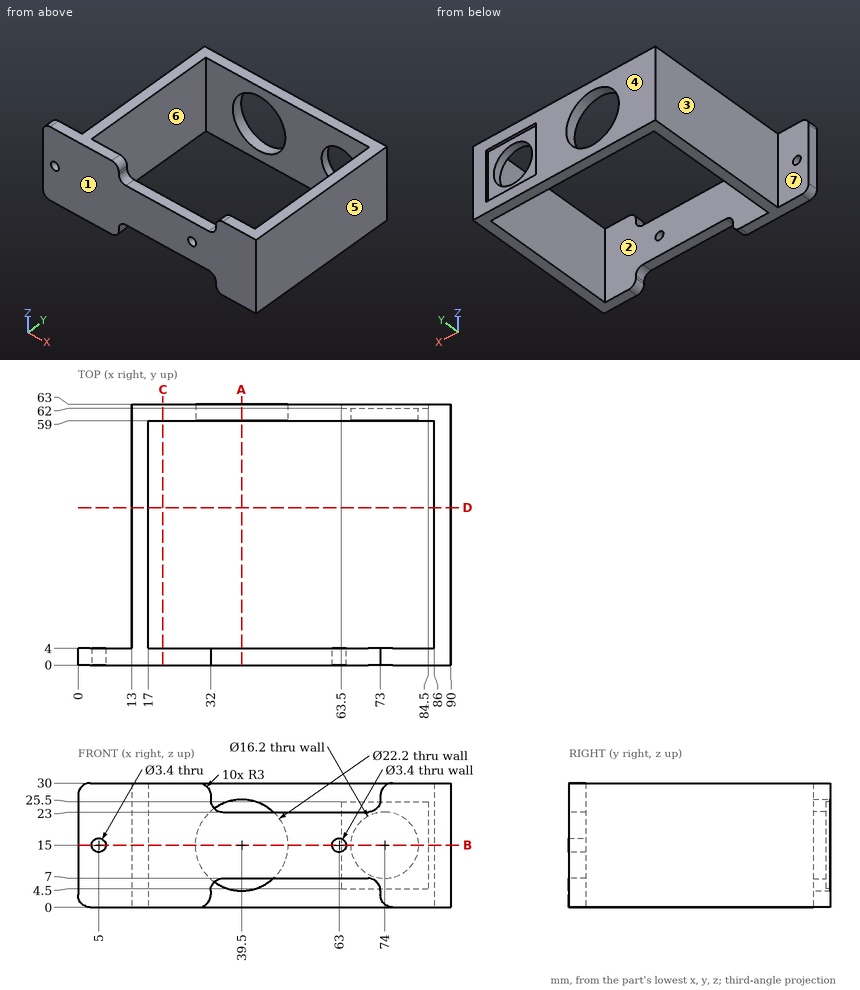
Here's the drawing with two shaded views (mm, measured from the low corner). I have some questions. A direction names the side the tool comes from. Coordinates: 2 decimals unless noted, no trailing zeros. Loops run counter-clockwise (first coordinate to the right, second up) from the corner with the lowest first, then second, coordinate; pieces in that order, holes last. Notation, with made-up numbers: (68, 70) -> (92, 70) arc R17 ccw to (92, 103) -> close; hole circle Ø3 at (65, 47.25). An arc over 180 degrees is marked (long way). Answer in a Markdown table with one row per item.
(1) Imagine slicing it at D-D (y = 38). List the corners of the cut face in (x, z) for me.
Results found:
| item | result |
|---|---|
| outline | (13, 0) -> (17, 0) -> (17, 30) -> (13, 30) -> close; (86, 0) -> (90, 0) -> (90, 30) -> (86, 30) -> close |
(2) Thinking about a two-plate mould opening in Y: for the marked faces 1, 2, 3 and 4, which applies, released by +Y, released by -Y, zero draft, split by the parting line, or undercut?
Results found:
| item | result |
|---|---|
| face 1 | released by -Y |
| face 2 | undercut |
| face 3 | zero draft |
| face 4 | released by +Y |
(3) For the marked faces 5, 6 and 7, which set-ups out of +Z, -Z, +X, -X, +Y, -Y let a thin tool reach every point of the face, with its end or its side?
Results found:
| item | result |
|---|---|
| face 5 | +Z, -Z, +X, +Y, -Y |
| face 6 | +Z, -Z |
| face 7 | +Z, -Z, -X, +Y |
(4) Imagine slicing it at C-C (x = 20.5). List the corners of the cut face in (y, z) for me.
Results found:
| item | result |
|---|---|
| outline | (0, 0) -> (4, 0) -> (4, 30) -> (0, 30) -> close; (59, 0) -> (63, 0) -> (63, 30) -> (59, 30) -> close |
(5) Will these pins go through, and if not, where does the flat tip stop? pin 1 Ø9 at (y, z) = (33, 15) entering from -X; pin 2 Ø1 at (x, z) = (63, 25.5) entering from -Y; pin 3 Ø2 at (x, y) = (49, 2) entering from +Z.
Results found:
| item | result |
|---|---|
| pin 1 | stops at x = 13 |
| pin 2 | stops at y = 59 |
| pin 3 | stops at z = 23 |
(6) If I drill on probe 1 along X at (y, z) = (2.35, 15); probe 2 along X at (y, z) = (60.3, 15); probe 3 along X at (y, z) = (57.5, 17.5), over which ranges is the centre line in solid material (lowest first)?
Results found:
| item | result |
|---|---|
| probe 1 | x = 0 to 3.3, 6.7 to 61.3, 64.7 to 90 |
| probe 2 | x = 13 to 28.4, 50.6 to 65.9, 82.1 to 90 |
| probe 3 | x = 13 to 17, 86 to 90 |
(7) Imagine slicing it at A-A (x = 39.5). List the corners of the cut face in (y, z) for me, plus the area to 3 significant figures.
Results found:
| item | result |
|---|---|
| outline | (0, 7) -> (4, 7) -> (4, 23) -> (0, 23) -> close; (59, 0) -> (63, 0) -> (63, 3.9) -> (59, 3.9) -> close; (59, 26.1) -> (63, 26.1) -> (63, 30) -> (59, 30) -> close |
| area | 95.2 mm^2 |
(8) Imagine slicing it at B-B (z = 15). Give the number of separate pieces and of enclosed holes in the cut face, plus the area to 3 significant figures.
Results found:
| item | result |
|---|---|
| separate pieces | 4 |
| enclosed holes | 0 |
| area | 922 mm^2 |
